Verification items for this drawing (mm, ordinates from the low corner). A direction names the side the tool comes from. Coordinates: 2 decimals unless noted, no trailing zeros. Order: outer loops, then holes, each group sorted by start corner. A loop starts at its lowest first (then second) coordinate and runs counter-clockwise, first axis right, second up. Notation, with made-up numbers: (75.25, 33.25) -> (122.25, 33.25) arc R10 cw to (122.25, 44.25) -> close; hole circle Ø10 at (83.5, 85). An arc over 180 degrees is marked (long way). Write item = value, one per line. Start each with the question number.
1. Set-up check for the marked faces 1 and 2: record each of +Z, -Z, +X, -X, +Y, -Y from which the full face is reachable in a straight line by a thin tool's end or side.
2. Cross-section at D-D on x = 27. Record the cut outline in (y, z).
3. Cross-section at B-B on x = 4.25. Record the cut outline in (y, z), plus the area to 3 significant figures.
4. Thickness scan on line 1 along Y through (x, z) = (37.75, 2.9); line 2 along X through (y, z) = (16.5, 4.75); line 3 along Y through (x, z) = (37.75, 1.05). Record the ranges inside material, lowest first. Write a range as from..to.
5. Cross-section at C-C on z = 1.35. Record the cut outline in (x, y), plus the area to 3 significant figures.
6. Go/stop test with flat-tipped pins: P1, Ø5, axis at x = 37.75, y = 14.6, coming from the +Z side; P2, Ø5.5, axis at x = 30, y = 11, coming from the +Z side; P3, Ø1, axis at x = 10.5, z = 3, coming from the -Y side. Record where each tip stops, or that it passes through.
7. Release check for a two-part mould opening along Y. For the marked faces 3, 4 and 5 record: +Y half, -Y half, draft (parallel to the pull), parting line (faces both ways), or undercut.
8. Cross-section at A-A on y = 4.4. Record the cut outline in (x, z), plus the area to 3 significant figures.
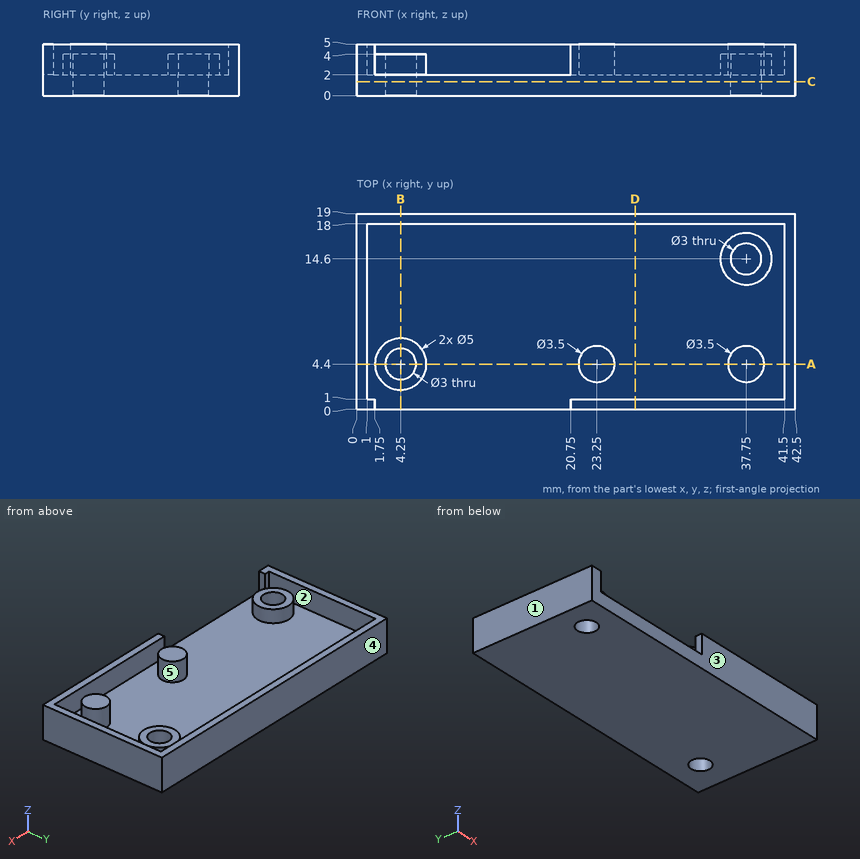
Worked out:
q1.face_1 = +Z, -Z, -X, +Y, -Y
q1.face_2 = +Z
q2.outline = (0, 0) -> (19, 0) -> (19, 5) -> (18, 5) -> (18, 2) -> (1, 2) -> (1, 5) -> (0, 5) -> close
q3.outline = (0, 0) -> (2.9, 0) -> (2.9, 4) -> (1.9, 4) -> (1.9, 2) -> (0, 2) -> close; (5.9, 0) -> (19, 0) -> (19, 5) -> (18, 5) -> (18, 2) -> (6.9, 2) -> (6.9, 4) -> (5.9, 4) -> close
q3.area = 39.0 mm²
q4.line_1 = 0..1, 2.65..6.15, 12.1..13.1, 16.1..17.1, 18..19
q4.line_2 = 0..1, 41.5..42.5
q4.line_3 = 0..13.1, 16.1..19
q5.outline = (0, 0) -> (42.5, 0) -> (42.5, 19) -> (0, 19) -> close; hole circle Ø3 at (4.25, 4.4); hole circle Ø3 at (37.75, 14.6)
q5.area = 793 mm²
q6.P1 = 4
q6.P2 = 2
q6.P3 = 18
q7.face_3 = -Y half
q7.face_4 = +Y half
q7.face_5 = undercut
q8.outline = (0, 0) -> (2.75, 0) -> (2.75, 4) -> (1.75, 4) -> (1.75, 2) -> (1, 2) -> (1, 5) -> (0, 5) -> close; (5.75, 0) -> (42.5, 0) -> (42.5, 5) -> (41.5, 5) -> (41.5, 2) -> (39.5, 2) -> (39.5, 5) -> (36, 5) -> (36, 2) -> (25, 2) -> (25, 5) -> (21.5, 5) -> (21.5, 2) -> (6.75, 2) -> (6.75, 4) -> (5.75, 4) -> close
q8.area = 110 mm²
